Check sheet for the modelled part. Datum: model origin and axes. Units: mm. Face numbers are marked on the shaded views. Round coordinates to 2 decimals unless told otherwise and drop trailing zeros. Loops run counter-clockwise (first coordinate to the right, second up) from the corner with the lowest first, then second, coordinate; pieces in that order, holes last. Notation, with made-up numbers: M 35,50.5 L 63,50.5 A17 cw 63,65.5 Z; hole C 61,49 d11. An arc over 180 degrees is marked long. One line per question, with ' | ' between items. Start each with the question number.
(1) Thickness scan on probe 1 along Z at (x, y) = (-34, 3.75); probe 2 along X at (y, z) = (8, -12.5); probe 3 along X at (y, z) = (6, -5). Record the ranges inside material, lowest first. Write a range as [from, to].
(2) Section check C-C (z = -12.7). Count the separate pieces of the cut face and the enclosed holes in it, and give its area (3 significant figures).
(3) Section check A-A (x = -19.05). Record the boundary of the cut face in (y, z).
(4) Section check B-B (x = 0). Record the boundary of the cut face in (y, z) (1 decimal), and give its area (3 significant figures).
(5) Go/stop test with flat-tipped pins: P1, Ø2.5, axis at x = 34.29, z = -12.7, coming from the -Y side; P2, Ø8, axis at x = -34.5, z = -10.5, coming from the +Y side. Record where each tip stops, or that it passes through.
(6) Draft check along X on the marked faces 1, 2 and 3. Enter one of: +X half, -X half, draft (parallel to the pull), parting line (faces both ways), or undercut.
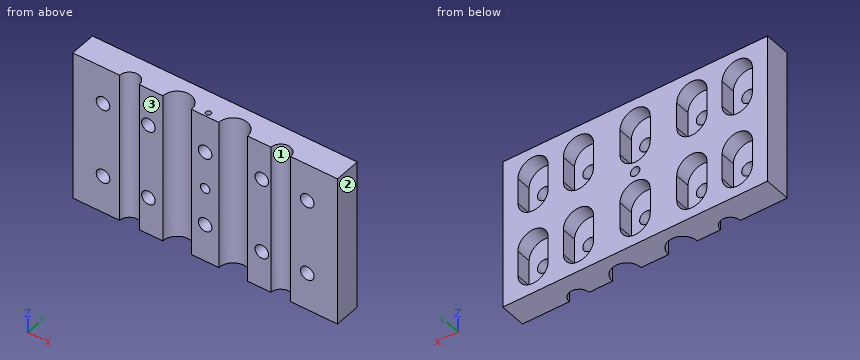
```python
from build123d import *

# Parameters (mm, degrees)
SKETCH1_W           = 88.9
SKETCH1_H           = 50.8
BOSS_EXTRUDE1_DEPTH = 8.89
SKETCH3_R           = 0.889
CUT_EXTRUDE3_DEPTH  = 9.652
CUT_EXTRUDE4_DEPTH  = 69.084319781
CUT_EXTRUDE5_DEPTH  = 69.084319781
CUT_EXTRUDE6_DEPTH  = 69.084319781
SKETCH2_R           = 2.286
CUT_EXTRUDE8_DEPTH  = 5.08
SKETCH11_R          = 2.286
CUT_EXTRUDE9_DEPTH  = 52.961472266
LPATTERN5_COUNT     = 2
LPATTERN5_PITCH     = 25.4
LPATTERN7_COUNT     = 2
LPATTERN7_PITCH     = 25.4
SKETCH12_R          = 1.5875
CUT_EXTRUDE10_DEPTH = 52.961472266
SKETCH13_R          = 0.889
CUT_EXTRUDE11_DEPTH = 9.652


with BuildPart() as part:
    # Sketch1 → Boss-Extrude1 (new body)
    with BuildSketch(Plane(origin=(0, 0, 0), x_dir=(1, 0, 0), z_dir=(0, 1, 0))):
        Rectangle(SKETCH1_W, SKETCH1_H)
    extrude(amount=BOSS_EXTRUDE1_DEPTH)

    # Sketch3 → Cut-Extrude3 (cut)
    with BuildSketch(Plane.XY.offset(25.4)):
        with Locations((6.35, 1.524)):
            Circle(SKETCH3_R)
    extrude(amount=-CUT_EXTRUDE3_DEPTH, mode=Mode.SUBTRACT)

    # Sketch4 → Cut-Extrude4 (cut, through all)
    with BuildSketch(Plane.XY.offset(25.4)):
        with BuildLine():
            Line((4.572, 0), (14.224, 0))
            ThreePointArc((14.224, 0), (9.398, 4.826), (4.572, 0))
        make_face()
    extrude(amount=-CUT_EXTRUDE4_DEPTH, mode=Mode.SUBTRACT)

    # Sketch5 → Cut-Extrude5 (cut, through all)
    with BuildSketch(Plane.XY.offset(25.4)):
        with BuildLine():
            Line((22.098, 0), (28.702, 0))
            ThreePointArc((28.702, 0), (25.4, 3.302), (22.098, 0))
        make_face()
    extrude(amount=-CUT_EXTRUDE5_DEPTH, mode=Mode.SUBTRACT)

    # Sketch6 → Cut-Extrude6 (cut, through all)
    with BuildSketch(Plane.XY.offset(25.4)):
        with BuildLine():
            Line((-28.702, 0), (-22.098, 0))
            ThreePointArc((-22.098, 0), (-25.4, 3.302), (-28.702, 0))
        make_face()
        with BuildLine():
            Line((-14.224, 0), (-4.572, 0))
            ThreePointArc((-4.572, 0), (-9.398, 4.826), (-14.224, 0))
        make_face()
    extrude(amount=-CUT_EXTRUDE6_DEPTH, mode=Mode.SUBTRACT)

    # Sketch2 → Cut-Extrude8 (cut)
    # profile 1 of 5: a face of its own
    with BuildSketch(Plane(origin=(0, 8.89, 0), x_dir=(1, 0, 0), z_dir=(0, 1, 0))):
        with BuildLine():
            Line((-29.21, 17.018), (-29.21, 8.382))
            ThreePointArc((-29.21, 8.382), (-34.29, 3.302), (-39.37, 8.382))
            Line((-39.37, 8.382), (-39.37, 17.018))
            ThreePointArc((-39.37, 17.018), (-34.29, 22.098), (-29.21, 17.018))
        make_face()
        with Locations(Location((-34.29, 12.7, 0), (0, 0, 270))):
            Circle(SKETCH2_R, mode=Mode.SUBTRACT)
    # profile 2 of 5: a face of its own
    with BuildSketch(Plane(origin=(0, 8.89, 0), x_dir=(1, 0, 0), z_dir=(0, 1, 0))):
        with BuildLine():
            Line((-13.97, 17.018), (-13.97, 8.382))
            ThreePointArc((-13.97, 8.382), (-19.05, 3.302), (-24.13, 8.382))
            Line((-24.13, 8.382), (-24.13, 17.018))
            ThreePointArc((-24.13, 17.018), (-19.05, 22.098), (-13.97, 17.018))
        make_face()
        with Locations(Location((-19.05, 12.7, 0), (0, 0, 270))):
            Circle(SKETCH2_R, mode=Mode.SUBTRACT)
    # profile 3 of 5: a face of its own
    with BuildSketch(Plane(origin=(0, 8.89, 0), x_dir=(1, 0, 0), z_dir=(0, 1, 0))):
        with BuildLine():
            Line((5.08, 17.018), (5.08, 8.382))
            ThreePointArc((5.08, 8.382), (0, 3.302), (-5.08, 8.382))
            Line((-5.08, 8.382), (-5.08, 17.018))
            ThreePointArc((-5.08, 17.018), (0, 22.098), (5.08, 17.018))
        make_face()
        with Locations(Location((0, 12.7, 0), (0, 0, 270))):
            Circle(SKETCH2_R, mode=Mode.SUBTRACT)
    # profile 4 of 5: a face of its own
    with BuildSketch(Plane(origin=(0, 8.89, 0), x_dir=(1, 0, 0), z_dir=(0, 1, 0))):
        with BuildLine():
            Line((24.13, 17.018), (24.13, 8.382))
            ThreePointArc((24.13, 8.382), (19.05, 3.302), (13.97, 8.382))
            Line((13.97, 8.382), (13.97, 17.018))
            ThreePointArc((13.97, 17.018), (19.05, 22.098), (24.13, 17.018))
        make_face()
        with Locations(Location((19.05, 12.7, 0), (0, 0, 270))):
            Circle(SKETCH2_R, mode=Mode.SUBTRACT)
    # profile 5 of 5: a face of its own
    with BuildSketch(Plane(origin=(0, 8.89, 0), x_dir=(1, 0, 0), z_dir=(0, 1, 0))):
        with BuildLine():
            Line((39.37, 17.018), (39.37, 8.382))
            ThreePointArc((39.37, 8.382), (34.29, 3.302), (29.21, 8.382))
            Line((29.21, 8.382), (29.21, 17.018))
            ThreePointArc((29.21, 17.018), (34.29, 22.098), (39.37, 17.018))
        make_face()
        with Locations(Location((34.29, 12.7, 0), (0, 0, 270))):
            Circle(SKETCH2_R, mode=Mode.SUBTRACT)
    cut_extrude8 = extrude(amount=-CUT_EXTRUDE8_DEPTH, mode=Mode.SUBTRACT)

    # Sketch11 → Cut-Extrude9 (cut, through all)
    with BuildSketch(Plane(origin=(0, 8.89, 0), x_dir=(1, 0, 0), z_dir=(0, 1, 0))):
        with Locations(Location((-34.29, 12.7, 0), (0, 0, 270))):
            Circle(SKETCH11_R)
        with Locations(Location((-19.05, 12.7, 0), (0, 0, 270))):
            Circle(SKETCH11_R)
        with Locations(Location((0, 12.7, 0), (0, 0, 270))):
            Circle(SKETCH11_R)
        with Locations(Location((19.05, 12.7, 0), (0, 0, 270))):
            Circle(SKETCH11_R)
        with Locations(Location((34.29, 12.7, 0), (0, 0, 270))):
            Circle(SKETCH11_R)
    cut_extrude9 = extrude(amount=-CUT_EXTRUDE9_DEPTH, mode=Mode.SUBTRACT)

    # LPattern5: Cut-Extrude8 ×2
    with Locations(*[(0, 0, i * LPATTERN5_PITCH) for i in range(1, LPATTERN5_COUNT)]):
        add(cut_extrude8, mode=Mode.SUBTRACT)

    # LPattern7: Cut-Extrude9 ×2
    with Locations(*[(0, 0, i * LPATTERN7_PITCH) for i in range(1, LPATTERN7_COUNT)]):
        add(cut_extrude9, mode=Mode.SUBTRACT)

    # Sketch12 → Cut-Extrude10 (cut, through all)
    with BuildSketch(Plane(origin=(0, 8.89, 0), x_dir=(1, 0, 0), z_dir=(0, 1, 0))):
        with Locations(Location((0, 0, 0), (0, 0, 270))):
            Circle(SKETCH12_R)
    extrude(amount=-CUT_EXTRUDE10_DEPTH, mode=Mode.SUBTRACT)

    # Sketch13 → Cut-Extrude11 (cut)
    with BuildSketch(Plane.XY.offset(25.4)):
        with Locations((0, 1.524)):
            Circle(SKETCH13_R)
    extrude(amount=-CUT_EXTRUDE11_DEPTH, mode=Mode.SUBTRACT)


solid = part.part
```
The answers:
1) probe 1: [-25.4, -14.97], [-10.43, 10.43], [14.97, 25.4] | probe 2: [-44.45, -39.37], [-29.21, -24.13], [-13.97, -5.08], [5.08, 13.97], [24.13, 29.21], [39.37, 44.45] | probe 3: [-44.45, -38.08], [-30.5, -22.84], [-15.26, -3.79], [3.79, 15.26], [22.84, 30.5], [38.08, 44.45]
2) separate pieces: 6 | enclosed holes: 0 | area: 338 mm²
3) outline: M 0,-25.4 L 8.89,-25.4 L 8.89,-22.1 L 3.81,-22.1 L 3.81,-14.99 L 0,-14.99 Z; M 0,-10.41 L 3.81,-10.41 L 3.81,-3.3 L 8.89,-3.3 L 8.89,3.3 L 3.81,3.3 L 3.81,10.41 L 0,10.41 Z; M 0,14.99 L 3.81,14.99 L 3.81,22.1 L 8.89,22.1 L 8.89,25.4 L 0,25.4 Z
4) outline: M 0,-25.4 L 8.9,-25.4 L 8.9,-22.1 L 3.8,-22.1 L 3.8,-15 L 0,-15 Z; M 0,-10.4 L 3.8,-10.4 L 3.8,-3.3 L 8.9,-3.3 L 8.9,-1.6 L 0,-1.6 Z; M 0,1.6 L 8.9,1.6 L 8.9,3.3 L 3.8,3.3 L 3.8,10.4 L 0,10.4 Z; M 0,15 L 3.8,15 L 3.8,22.1 L 8.9,22.1 L 8.9,25.4 L 2.4,25.4 L 2.4,15.7 L 0.6,15.7 L 0.6,25.4 L 0,25.4 Z | area: 180 mm²
5) P1: through | P2: y = 3.81
6) face 1: undercut | face 2: +X half | face 3: draft
